Geometry check sheet. Reference: the model listing, model coordinates, mm. Face numbers are marked on the shaded views. A direction names the side the tool comes from. Coordinates: 2 decimals unless noted, no trailing zeros. Order: outer loops, then holes, each group sorted by start corner. A loop starts at its lowest first (then second) coordinate and runs counter-clockwise, first axis right, second up.
Autodesk Inventor part; units mm, degrees
ref_plane "YZ Plane" through (0, 0, 0) normal (1, 0, 0) x (0, 1, 0)
ref_plane "XZ Plane" through (0, 0, 0) normal (0, 1, 0) x (-1, 0, 0)
ref_plane "XY Plane" through (0, 0, 0) normal (0, 0, 1) x (1, 0, 0)
sketch "Sketch1" plane through (0, 0, 0) normal (0, 1, 0) x (-1, 0, 0)
  line L0 (55, -18) -> (-55, -18)
  line L1 (-55, -18) -> (-55, 18)
  line L2 (-55, 18) -> (55, 18)
  line L3 (55, 18) -> (55, -18)
  line L4 (55, -18) -> (-55, 18) construction
  line L5 (-55, -18) -> (55, 18) construction
  point P0 (0, 0)
  dimension "d0" = 110
  dimension "d1" = 36
extrude "Body" add sketch "Sketch1" along normal mid plane 4.5
ref_plane "Work Plane4" through (0, 0.75, 0) normal (0, 1, 0) x (1, 0, 0)
sketch "Sketch6" plane through (0, 0.75, 0) normal (0, 1, 0) x (1, 0, 0)
  line L0 (-30.5, 7) -> (30.5, 7)
  line L1 (30.5, 7) -> (30.5, -7)
  line L2 (30.5, -7) -> (-30.5, -7)
  line L3 (-30.5, -7) -> (-30.5, 7)
  line L4 (-30.5, 7) -> (30.5, -7) construction
  line L5 (30.5, 7) -> (-30.5, -7) construction
  point P0 (0, 0)
  dimension "d15" = 61
  dimension "d16" = 14
extrude "Flow Volume" cut sketch "Sketch6" along normal through all both and the other way through all
sketch "Sketch14" plane through (0, 2.25, 0) normal (0, 1, 0) x (1, 0, 0)
  line L0 (38.5, 18) -> (38.5, -18)
  line L1 (38.5, 0) -> (55, 0)
  line L2 (55, 18) -> (55, -18)
  circle A0 centre (42, 0) radius 3.5
  point P0 (0, 0)
  dimension "d37" = 7
extrude "Inlet" add sketch "Sketch14" along normal blind 22
sketch "Sketch15" plane through (42, 24.25, 0) normal (0, 1, 0) x (1, 0, 0)
  circle A0 centre (0, 0) radius 1.5
  circle A1 centre (0, 0) radius 3.5
  point P0 (-42, 0)
  dimension "d40" = 3
extrude "Inlet Hole" cut sketch "Sketch15" against normal through all contours A0
ref_plane "Work Plane1" through (0, 0.75, 18) normal (-1, 0, 0) x (0, 0, -1)
mirror "Outlet" about plane through (0, 0.75, 18) normal (-1, 0, 0) of "Inlet", "Inlet Hole"
sketch "Sketch22" plane through (0, -2.25, 0) normal (0, -1, 0) x (1, 0, 0)
  line L0 (-42.5, -13) -> (42.5, -13)
  line L1 (47.5, -8) -> (47.5, 8)
  line L2 (42.5, 13) -> (-42.5, 13)
  line L3 (-47.5, 8) -> (-47.5, -8)
  line L4 (-47.5, -13) -> (47.5, 13) construction
  line L5 (47.5, -13) -> (-47.5, 13) construction
  line L6 (-42.5, -13.5) -> (42.5, -13.5)
  line L7 (48, -8) -> (48, 8)
  line L8 (42.5, 13.5) -> (-42.5, 13.5)
  line L9 (-48, 8) -> (-48, -8)
  line L10 (-48, -13.5) -> (48, 13.5) construction
  line L11 (48, -13.5) -> (-48, 13.5) construction
  arc A0 (-47.5, -8) -> (-42.5, -13) centre (-42.5, -8) ccw
  arc A1 (42.5, -13) -> (47.5, -8) centre (42.5, -8) ccw
  arc A2 (47.5, 8) -> (42.5, 13) centre (42.5, 8) ccw
  arc A3 (-42.5, 13) -> (-47.5, 8) centre (-42.5, 8) ccw
  arc A4 (-48, -8) -> (-42.5, -13.5) centre (-42.5, -8) ccw
  arc A5 (42.5, -13.5) -> (48, -8) centre (42.5, -8) ccw
  arc A6 (48, 8) -> (42.5, 13.5) centre (42.5, 8) ccw
  arc A7 (-42.5, 13.5) -> (-48, 8) centre (-42.5, 8) ccw
  point P0 (0, 0)
  dimension "d56" = 95
  dimension "d57" = 26
  dimension "d58" = 0.5
  dimension "d59" = 0.5
  dimension "d60" = 5
  dimension "d61" = 5.5
extrude "Knife Edge" add sketch "Sketch22" along normal blind 1
sketch "Sketch23" plane through (0, -2.25, 0) normal (0, -1, 0) x (1, 0, 0)
  line L0 (38.5, 13) -> (-38.5, 13)
  line L1 (-38.5, 13) -> (-38.5, -13)
  line L2 (-38.5, -13) -> (38.5, -13)
  line L3 (38.5, -13) -> (38.5, 13)
  line L4 (38.5, 13) -> (-38.5, -13) construction
  line L5 (-38.5, 13) -> (38.5, -13) construction
  line L6 (-42.5, -13) -> (42.5, -13)
  point P0 (0, 0)
  dimension "d64" = 77
extrude "Extrusion14" cut sketch "Sketch23" against normal blind 1.5
properties part number "Top 6_7"
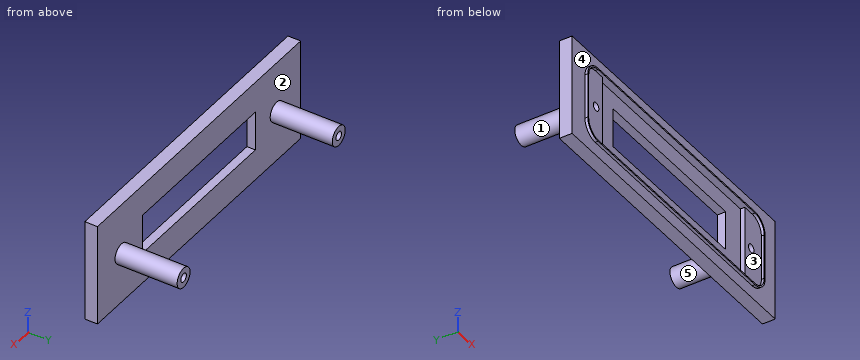
Item 1: Sectioned sample at B-B (x = -1). Record the cut outline in (y, z).
Item 2: Sectioned sample at A-A (y = 0.25). Record the cut outline in (x, z).
Item 3: Tool access check on the marked faces 4 and 5. Record the directions out of +Z, -Z, +X, -X, +Y, -Y that give a thin tool (end or side, any length) a straight path to the whole face; none if there is none.
Item 4: Sectioned sample at D-D (y = 6.25). Record the cut outline in (x, z), and give its area (3 significant figures).
Item 5: Depth check by flat-ended pin: P1, Ø0.5, axis at y = -3, z = -1, coming from the -X side; P2, Ø5, axis at x = -10, z = -6.5, coming from the -Y side; P3, Ø10, axis at y = 20.5, z = 7, coming from the +X side. Enter the tip coordinate at first touch or a pass-through.
Item 6: Release check for a two-part mould opening along Z. For the marked faces 1, 2 and 3 record: pulls with the +Z half, pulls with the -Z half, needs draft (parallel to the pull), parting line crosses it, or undercut.
Item 7: Thickness scan on line 1 along X through (y, z) = (13.75, 0); line 2 along X through (y, z) = (15.25, 1); line 3 along Z through (x, y) = (-1, 0). Record the ranges inside material, lowest first.
Item 8: Sectioned sample at C-C (x = -37.5). Record the cut outline in (y, z), and give its area (3 significant figures).
Geometry check:
1. outline: (-3.25, -13.5) - (-2.25, -13.5) - (-2.25, -18) - (2.25, -18) - (2.25, -7) - (-0.75, -7) - (-0.75, -13) - (-3.25, -13) - close; (-3.25, 13) - (-0.75, 13) - (-0.75, 7) - (2.25, 7) - (2.25, 18) - (-2.25, 18) - (-2.25, 13.5) - (-3.25, 13.5) - close
2. outline: (-55, -18) - (55, -18) - (55, 18) - (-55, 18) - close; hole circle Ø3 at (-42, 0); hole (-30.5, -7) - (30.5, -7) - (30.5, 7) - (-30.5, 7) - close; hole circle Ø3 at (42, 0)
3. face 4: -Y
3. face 5: +Y
4. outline: circle Ø7 at (-42, 0); circle Ø7 at (42, 0); hole circle Ø3 at (-42, 0); hole circle Ø3 at (42, 0)
4. area: 62.8 mm2
5. P1: stops at x = -48
5. P2: stops at y = -0.75
5. P3: stops at x = 44.87
6. face 1: parting line crosses it
6. face 2: needs draft
6. face 3: undercut
7. line 1: x = -45.5 to -43.5, -40.5 to -38.5, 38.5 to 40.5, 43.5 to 45.5
7. line 2: x = -45.35 to -43.12, -40.88 to -38.65, 38.65 to 40.88, 43.12 to 45.35
7. line 3: z = -18 to -7, 7 to 18
8. outline: (-3.25, -13.5) - (-2.25, -13.5) - (-2.25, -18) - (2.25, -18) - (2.25, 18) - (-2.25, 18) - (-2.25, 13.5) - (-3.25, 13.5) - (-3.25, 13) - (-0.75, 13) - (-0.75, -13) - (-3.25, -13) - close
8. area: 124 mm2
